Here's how the part is built. I have some questions about the finished solid (model axes, mm). Face numbers are marked on the shaded views. A direction names the side the tool comes from. Give positions to 0.01 mm unless a question says otherwise; leave off trailing zeros. Loops run counter-clockwise (first coordinate to the right, second up) from the corner with the lowest first, then second, coordinate; pieces in that order, holes last. Notation, with made-up numbers: (82.25, 9.25) -> (140.25, 9.25) arc R16 cw to (140.25, 20.25) -> close; hole circle Ø4 at (-6, 58). An arc over 180 degrees is marked (long way). Answer in a Markdown table with one row per item. Add a question column.
Item 1: For P1, Ø2, axis at x = 6.5, z = 1.5, coming from the +Y side; P2, Ø6, axis at y = 18.5, z = 10.5, coming from the -X side; P3, Ø1.2, axis at x = 0, z = -4.17, coming from the +Y side, each with a flat end and sliding along its axis, tell me the tip position at first contact or that it passes through.
Item 2: If we section it at B-B (z = -10.5): Write out the boundary of the cut face in (x, y).
Item 3: Which directions (+Z, -Z, +X, -X, +Y, -Y) give clear straight access to the entire face, cutting with the end or side of a thin tool? Please do the marked faces 1, 2 and 3.
Item 4: If we section it at D-D (y = 89): Write out the boundary of the cut face in (x, z), then the cut area to 3 significant figures.
Item 5: If we section it at A-A (y = 36): Write out the boundary of the cut face in (x, z).
Item 6: If I drill on line 1 (Y direction, x = -2.5, z = 16); line 2 (Y direction, x = -1, z = -14); line 3 (Y direction, x = -2, z = -11.5), over which ranges is the centre line in solid material (lowest first)?
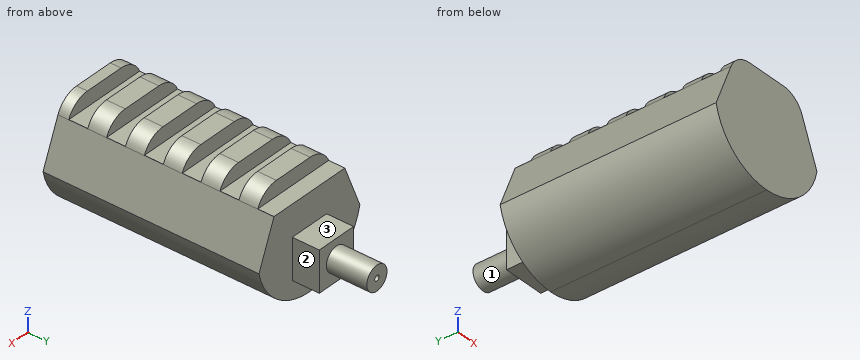
```python
from build123d import *

# Parameters (mm, degrees)
BOSS_EXTRUDE1_DEPTH     = 80
BOSS_EXTRUDE2_DEPTH     = 5
BOSS_EXTRUDE3_START     = 75
BOSS_EXTRUDE3_DEPTH     = 5
CUT_EXTRUDE1_START      = 20
SKETCH2_W               = 31.64103086
SKETCH2_H               = 7
SKETCH2_H_2             = 6
CUT_EXTRUDE1_DEPTH      = 5.5
CROQUIS1_W              = 15.3
CROQUIS1_H              = 15
SALIENTE_EXTRUIR1_DEPTH = 10
CROQUIS2_R              = 4.5
CROQUIS2_R_2            = 1
SALIENTE_EXTRUIR2_DEPTH = 15
CORTAR_EXTRUIR1_START   = -24
CROQUIS2_2_R            = 1
CORTAR_EXTRUIR1_DEPTH   = 24


# Read off the part's stored shape, not the designer's step: Boss-Extrude3
with BuildPart() as part:
    # Sketch1 → Boss-Extrude1 (new body)
    with BuildSketch(Plane(origin=(0, 0, 0), x_dir=(1, 0, 0), z_dir=(0, 1, 0))):
        with BuildLine():
            Line((7.5, -20), (-7.5, -20))
            ThreePointArc((-7.5, -20), (-12.50622569, -18.479151312), (-15.82051543, -14.430600965))
            Line((-15.82051543, -14.430600965), (-22.5, 1.769696007))
            ThreePointArc((-22.5, 1.769696007), (-14.479243624, 14.870408615), (0, 20))
            ThreePointArc((0, 20), (14.479243624, 14.870408615), (22.5, 1.769696007))
            Line((22.5, 1.769696007), (15.82051543, -14.430600965))
            ThreePointArc((15.82051543, -14.430600965), (12.50622569, -18.479151312), (7.5, -20))
        make_face()
        with BuildLine():
            Line((-7.5, -13), (7.5, -13))
            ThreePointArc((7.5, -13), (11.393731092, -11.817117687), (13.971512001, -8.668245195))
            Line((13.971512001, -8.668245195), (15.06741388, -6.010265271))
            ThreePointArc((15.06741388, -6.010265271), (0, 16.5), (-15.06741388, -6.010265271))
            Line((-15.06741388, -6.010265271), (-13.971512001, -8.668245195))
            ThreePointArc((-13.971512001, -8.668245195), (-11.393731092, -11.817117687), (-7.5, -13))
        make_face(mode=Mode.SUBTRACT)
    extrude(amount=BOSS_EXTRUDE1_DEPTH)

    # Sketch1<2> → Boss-Extrude2 (add)
    with BuildSketch(Plane(origin=(0, 0, 0), x_dir=(1, 0, 0), z_dir=(0, 1, 0))):
        with BuildLine():
            ThreePointArc((-13.971512001, -8.668245195), (-11.393731092, -11.817117687), (-7.5, -13))
            Line((-7.5, -13), (7.5, -13))
            ThreePointArc((7.5, -13), (11.393731092, -11.817117687), (13.971512001, -8.668245195))
            Line((13.971512001, -8.668245195), (15.06741388, -6.010265271))
            ThreePointArc((15.06741388, -6.010265271), (0, 16.5), (-15.06741388, -6.010265271))
            Line((-15.06741388, -6.010265271), (-13.971512001, -8.668245195))
        make_face()
    extrude(amount=BOSS_EXTRUDE2_DEPTH)

    # Boss-Extrude3 outline → Boss-Extrude3 (add)
    with BuildSketch(Plane(origin=(0, 0, 0), x_dir=(1, 0, 0), z_dir=(0, 1, 0)).offset(BOSS_EXTRUDE3_START)):
        with BuildLine():
            Line((-15.06741388, -6.010265271), (-13.971512001, -8.668245195))
            ThreePointArc((-13.971512001, -8.668245195), (-11.393731092, -11.817117687), (-7.5, -13))
            Line((-7.5, -13), (7.5, -13))
            ThreePointArc((7.5, -13), (11.393731092, -11.817117687), (13.971512001, -8.668245195))
            Line((13.971512001, -8.668245195), (15.06741388, -6.010265271))
            ThreePointArc((15.06741388, -6.010265271), (0, 16.5), (-15.06741388, -6.010265271))
        make_face()
    extrude(amount=BOSS_EXTRUDE3_DEPTH)

    # Sketch2 → Cut-Extrude1 (cut)
    with BuildSketch(Plane.XY.offset(CUT_EXTRUDE1_START)):
        with Locations((0, 7.5)):
            Rectangle(SKETCH2_W, SKETCH2_H)
        with Locations((0, 21.5)):
            Rectangle(SKETCH2_W, SKETCH2_H)
        with Locations((0, 35.5)):
            Rectangle(SKETCH2_W, SKETCH2_H)
        with Locations((0, 49.5)):
            Rectangle(SKETCH2_W, SKETCH2_H)
        with Locations((0, 63.5)):
            Rectangle(SKETCH2_W, SKETCH2_H)
        with Locations((0, 77)):
            Rectangle(SKETCH2_W, SKETCH2_H_2)
    extrude(amount=-CUT_EXTRUDE1_DEPTH, mode=Mode.SUBTRACT)

    # Croquis1 → Saliente-Extruir1 (add)
    with BuildSketch(Plane(origin=(0, 80, 0), x_dir=(1, 0, 0), z_dir=(0, 1, 0))):
        with Locations((0, 4.5)):
            Rectangle(CROQUIS1_W, CROQUIS1_H)
    extrude(amount=SALIENTE_EXTRUIR1_DEPTH)

    # Croquis2 → Saliente-Extruir2 (add)
    with BuildSketch(Plane(origin=(0, 90, 0), x_dir=(1, 0, 0), z_dir=(0, 1, 0))):
        with Locations(Location((0, 4.172752701, 0), (0, 0, 270))):
            Circle(CROQUIS2_R)
        with Locations(Location((0, 4.172752701, 0), (0, 0, 270))):
            Circle(CROQUIS2_R_2, mode=Mode.SUBTRACT)
    extrude(amount=SALIENTE_EXTRUIR2_DEPTH)

    # Croquis2<2> → Cortar-Extruir1 (cut)
    with BuildSketch(Plane(origin=(0, 90, 0), x_dir=(1, 0, 0), z_dir=(0, 1, 0)).offset(CORTAR_EXTRUIR1_START)):
        with Locations(Location((0, 4.172752701, 0), (0, 0, 90))):
            Circle(CROQUIS2_2_R)
    extrude(amount=CORTAR_EXTRUIR1_DEPTH, mode=Mode.SUBTRACT)


solid = part.part
```
Recorded:
| question | item | result |
|---|---|---|
| 1 | P1 | stops at y = 90 |
| 1 | P2 | stops at x = -18.68 |
| 1 | P3 | stops at y = 5 |
| 2 | outline | (-18.62, 0) -> (18.62, 0) -> (18.62, 80) -> (7.65, 80) -> (7.65, 90) -> (-7.65, 90) -> (-7.65, 80) -> (-18.62, 80) -> close; hole (-12.63, 5) -> (12.63, 5) -> (12.63, 75) -> (-12.63, 75) -> close |
| 3 | face 1 | +Y |
| 3 | face 2 | +Z, -Z, +X, +Y |
| 3 | face 3 | +Z, +X, -X, +Y |
| 4 | outline | (-7.65, -12) -> (7.65, -12) -> (7.65, 3) -> (-7.65, 3) -> close; hole circle Ø2 at (0, -4.17) |
| 4 | area | 226 mm^2 |
| 5 | outline | (-22.5, -1.77) arc R23 ccw to (22.5, -1.77) -> (15.82, 14.43) arc R9 ccw to (15.79, 14.5) -> (-15.79, 14.5) arc R9 ccw to (-15.82, 14.43) -> close; hole (-15.07, 6.01) arc R16.3 ccw (long way) to (15.07, 6.01) -> (13.97, 8.67) arc R7 ccw to (7.5, 13) -> (-7.5, 13) arc R7 ccw to (-13.97, 8.67) -> close |
| 6 | line 1 | y = 0 to 4, 11 to 18, 25 to 32, 39 to 46, 53 to 60, 67 to 74 |
| 6 | line 2 | y = 0 to 5, 75 to 80 |
| 6 | line 3 | y = 0 to 5, 75 to 90 |
